```python
from build123d import *

# Parameters (mm, degrees)
SKETCH1_W           = 1205
SKETCH1_H           = 805
BOSS_EXTRUDE1_DEPTH = 19
SKETCH2_R           = 27.5
BOSS_EXTRUDE2_DEPTH = 696
FILLET1_R           = 60


with BuildPart() as part:
    # Sketch1 → Boss-Extrude1 (new body)
    with BuildSketch(Plane(origin=(0, 0, 0), x_dir=(1, 0, 0), z_dir=(0, 1, 0))):
        Rectangle(SKETCH1_W, SKETCH1_H)
    extrude(amount=BOSS_EXTRUDE1_DEPTH)

    # Sketch2 → Boss-Extrude2 (add)
    with BuildSketch(Plane(origin=(0, 0, 0), x_dir=(-1, 0, 0), z_dir=(0, -1, 0))):
        with Locations(Location((546, 346, 0), (0, 0, 270))):
            Circle(SKETCH2_R)
        with Locations(Location((-544.120521212, 346, 0), (0, 0, 270))):
            Circle(SKETCH2_R)
        with Locations(Location((-546, -347.089225584, 0), (0, 0, 270))):
            Circle(SKETCH2_R)
        with Locations(Location((546, -346, 0), (0, 0, 270))):
            Circle(SKETCH2_R)
    extrude(amount=BOSS_EXTRUDE2_DEPTH)

    # Fillet1
    fillet1_edges = [part.edges().sort_by_distance(p)[0] for p in [
        (-602.5, 9.5, -402.5),
        (-602.5, 9.5, 402.5),
        (602.5, 9.5, 402.5),
        (602.5, 9.5, -402.5),
    ]]
    fillet(fillet1_edges, radius=FILLET1_R)


solid = part.part
```
Source: CAD feature listing. Evaluate the final solid. Frame: model axes, mm. A direction names the side the tool comes from. Coordinates: 2 decimals unless noted, no trailing zeros. Loops run counter-clockwise (first coordinate to the right, second up) from the corner with the lowest first, then second, coordinate; pieces in that order, holes last. Notation, with made-up numbers: M 37,-10.5 L 73,-10.5 A6 cw 73,-6.5 Z; hole C 74.25,0 d10. An arc over 180 degrees is marked long. Put each result on its own line as item: value. Start each with the question number.
1) Ray query, L1, parallel to Y at x = -467, z = -1; L2, parallel to X at y = -204.5, z = -323; L3, parallel to X at y = -585.5, z = -321.5. Return the intervals inside material, ascending. Write a range as from..to.
2) Cut plane A-A on x = -18. Return the cut outline in (y, z), then the cut area to 3 significant figures.
3) Cut plane B-B on z = 104. Return the cut outline in (x, y).
4) Reachability of faces 1 (the face through (518.734, -343.128, 343.509)), 2 (the face through (-546, -696, -346)) from +Z, -Z, +X, -X, +Y, -Y: full face, straight path, thin tool, end or side. Return the list, or none.
5) Cut plane C-C on y = -179. Return the cut outline in (x, z).
6) Pull-direction query (X, two-part tool) for faces 3 (the face through (-569.19, -343.13, 360.78)), 4 (the face through (544, -696, -346)), 5 (the face through (584.46, 9.63, 385.39)); classes: pulls with the +X half, pulls with the -X half, needs draft (parallel to the pull), parting line crosses it, or undercut.
The answers:
1. L1: y = 0..19
1. L2: x = -561.07..-530.93, 529.05..559.2
1. L3: x = -558.49..-533.51, 531.63..556.61
2. outline: M 0,-402.5 L 19,-402.5 L 19,402.5 L 0,402.5 Z
2. area: 15,300 mm²
3. outline: M -602.5,0 L 602.5,0 L 602.5,19 L -602.5,19 Z
4. face 1: -Y
4. face 2: +Z, -Z, +X, -X, -Y
5. outline: C -546,-346 d55; C -546,346 d55; C 544.12,-346 d55; C 546,347.09 d55
6. face 3: undercut
6. face 4: needs draft
6. face 5: pulls with the +X half
